Geometry: final body of the model. Coordinates: model frame, mm. A direction names the side the tool comes from. Round coordinates to 2 decimals unless told otherwise and drop trailing zeros. Loops run counter-clockwise (first coordinate to the right, second up) from the corner with the lowest first, then second, coordinate; pieces in that order, holes last. Notation, with made-up numbers: (81, 21) -> (109, 21) arc R13 ccw to (109, 33) -> close; hole circle Ø1 at (54, 27.25). An arc over 180 degrees is marked (long way). Answer in a Markdown table with one row per item.
```python
from build123d import *

# Parameters (mm, degrees)
SCHIZZO1_R                   = 3.1
SCHIZZO1_R_2                 = 1.75
ESTRUSIONE_ESTRUSIONE1_DEPTH = 5


with BuildPart() as part:
    # Schizzo1 → Estrusione-Estrusione1 (new body)
    with BuildSketch(Plane.XY):
        with BuildLine():
            Line((0, 0), (0, 449))
            Line((0, 449), (171.5, 449))
            ThreePointArc((171.5, 449), (173.621320344, 448.121320344), (174.5, 446))
            Line((174.5, 446), (174.5, 417))
            ThreePointArc((174.5, 417), (177.428932188, 409.928932188), (184.5, 407))
            Line((184.5, 407), (264.5, 407))
            ThreePointArc((264.5, 407), (271.571067812, 409.928932188), (274.5, 417))
            Line((274.5, 417), (274.5, 446))
            ThreePointArc((274.5, 446), (275.378679656, 448.121320344), (277.5, 449))
            Line((277.5, 449), (449, 449))
            Line((449, 449), (449, 0))
            Line((449, 0), (0, 0))
        make_face()
        with Locations((11.5, 11.5)):
            Circle(SCHIZZO1_R, mode=Mode.SUBTRACT)
        with Locations((437.5, 11.5)):
            Circle(SCHIZZO1_R, mode=Mode.SUBTRACT)
        with Locations((437.5, 437.5)):
            Circle(SCHIZZO1_R, mode=Mode.SUBTRACT)
        with Locations((11.5, 437.5)):
            Circle(SCHIZZO1_R, mode=Mode.SUBTRACT)
        with Locations((309.5, 424)):
            Circle(SCHIZZO1_R_2, mode=Mode.SUBTRACT)
        with BuildLine():
            Line((344.715899345, 434), (405.440355678, 434))
            ThreePointArc((405.440355678, 434), (415.440355678, 424), (405.440355678, 414))
            Line((405.440355678, 414), (344.715899345, 414))
            ThreePointArc((344.715899345, 414), (334.715899345, 424), (344.715899345, 434))
        make_face(mode=Mode.SUBTRACT)
    extrude(amount=ESTRUSIONE_ESTRUSIONE1_DEPTH)


solid = part.part
```
Item 1: Pin query (flat end, axial travel): pin 1 Ø4.5 at (x, y) = (309.5, 424) entering from -Z; pin 2 Ø3.5 at (x, y) = (437.5, 11.5) entering from +Z. Return the tip coordinate at first contact, or that it passes through.
Answer:
| item | result |
|---|---|
| pin 1 | stops at z = 0 |
| pin 2 | passes through |
Item 2: Cut plane A-A (z = 1.2). Output: boundary loops of the cut face in (x, y).
Answer:
| item | result |
|---|---|
| outline | (0, 0) -> (449, 0) -> (449, 449) -> (277.5, 449) arc R3 ccw to (274.5, 446) -> (274.5, 417) arc R10 cw to (264.5, 407) -> (184.5, 407) arc R10 cw to (174.5, 417) -> (174.5, 446) arc R3 ccw to (171.5, 449) -> (0, 449) -> close; hole circle Ø6.2 at (11.5, 11.5); hole circle Ø6.2 at (11.5, 437.5); hole circle Ø3.5 at (309.5, 424); hole (344.72, 414) -> (405.44, 414) arc R10 ccw to (405.44, 434) -> (344.72, 434) arc R10 ccw to start; hole circle Ø6.2 at (437.5, 11.5); hole circle Ø6.2 at (437.5, 437.5) |
Item 3: Draft query along X for faces 1 (the face through (228, 228, 0)), 2 (the face through (415.438, 424.22, 2.465)). Return one class per face: pulls with the +X half, pulls with the -X half, needs draft (parallel to the pull), parting line crosses it, or undercut.
Answer:
| item | result |
|---|---|
| face 1 | needs draft |
| face 2 | undercut |
Item 4: Line query: probe 1 along X at (y, z) = (437.5, 2.4); probe 2 along Y at (x, z) = (11.5, 1.5); probe 3 along X at (y, z) = (424, 3.1). Output: solid intervals per line, ascending. Write a range as [from, to].
Answer:
| item | result |
|---|---|
| probe 1 | x = [0, 8.4], [14.6, 174.5], [274.5, 434.4], [440.6, 449] |
| probe 2 | y = [0, 8.4], [14.6, 434.4], [440.6, 449] |
| probe 3 | x = [0, 174.5], [274.5, 307.75], [311.25, 334.72], [415.44, 449] |
Item 5: Reachability of faces 3 (the face through (271.49, 409.85, 2.46)), 4 (the face through (228, 228, 5)), 5 (the face through (334.72, 423.78, 2.46)) from +Z, -Z, +X, -X, +Y, -Y: full face, straight path, thin tool, end or side. Return the list, or none.
Answer:
| item | result |
|---|---|
| face 3 | +Z, -Z, +Y |
| face 4 | +Z, +X, -X, +Y, -Y |
| face 5 | +Z, -Z |
